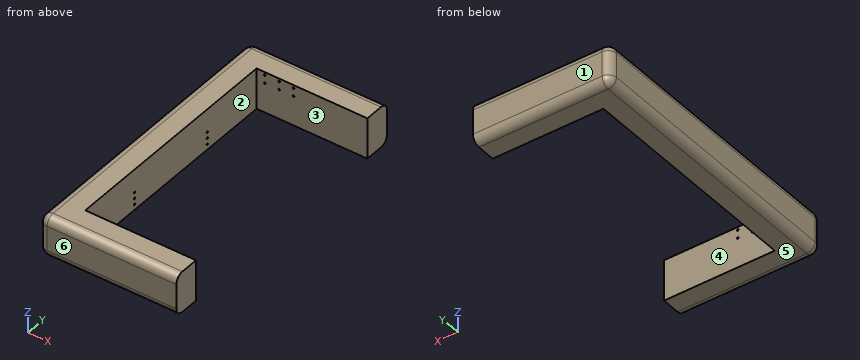
Autodesk Inventor part; units mm, degrees
ref_plane "YZ Plane" through (0, 0, 0) normal (1, 0, 0) x (0, 1, 0)
ref_plane "XZ Plane" through (0, 0, 0) normal (0, 1, 0) x (-1, 0, 0)
ref_plane "XY Plane" through (0, 0, 0) normal (0, 0, 1) x (1, 0, 0)
sketch "Sketch1" plane through (0, 0, 0) normal (0, 0, 1) x (1, 0, 0)
  line L0 (0, 0) -> (0, 719.074)
  line L1 (0, 719.074) -> (342.9, 719.074)
  line L2 (0, 0) -> (342.9, 0)
  line L3 (342.9, 801.624) -> (-82.55, 801.624)
  line L4 (-82.55, 801.624) -> (-82.55, -82.55)
  line L5 (-82.55, -82.55) -> (342.9, -82.55)
  line L6 (342.9, 719.074) -> (342.9, 801.624)
  line L7 (342.9, 0) -> (342.9, -82.55)
  dimension "d0" = 719.074
  dimension "d1" = 342.9
  dimension "d2" = 82.55
extrude "Extrusion1" add sketch "Sketch1" along normal blind 127
fillet "Fillet1" radius 25.4 8 edges at (130.175, 801.624, 127) (130.175, 801.624, 0) (-82.55, 801.624, 63.5) (-82.55, 359.537, 127) (-82.55, 359.537, 0) (-82.55, -82.55, 63.5) (130.175, -82.55, 0) (130.175, -82.55, 127)
sketch "Sketch2" plane through (0, 719.074, 0) normal (0, -1, 0) x (1, 0, 0)
  line L0 (342.9, 0) -> (342.9, 127) construction
  line L1 (0, 127) -> (342.9, 127) construction
  line L2 (342.9, 127) -> (114.3, 127) construction
  line L3 (114.3, 127) -> (69.85, 127) construction
  line L4 (69.85, 127) -> (25.4, 127) construction
  line L5 (114.3, 127) -> (114.3, 117.475) construction
  line L6 (114.3, 117.475) -> (69.85, 117.475) construction
  line L7 (69.85, 117.475) -> (25.4, 117.475) construction
  line L8 (25.4, 117.475) -> (25.4, 92.075) construction
  line L9 (25.4, 92.075) -> (69.85, 92.075) construction
  line L10 (69.85, 92.075) -> (114.3, 92.075) construction
  circle A0 centre (114.3, 117.475) radius 2.667
  circle A1 centre (69.85, 117.475) radius 2.667
  circle A2 centre (25.4, 117.475) radius 2.667
  circle A3 centre (25.4, 92.075) radius 2.667
  circle A4 centre (69.85, 92.075) radius 2.667
  circle A5 centre (114.3, 92.075) radius 2.667
  point P0 (0, 0)
  dimension "d7" = 228.6
  dimension "d8" = 44.45
  dimension "d9" = 44.45
  dimension "d10" = 9.525
  dimension "d11" = 25.4
  dimension "d12" = 5.334
extrude "Extrusion2" cut sketch "Sketch2" against normal blind 4.7625
sketch "Sketch3" plane through (0, 0, 0) normal (0, 1, 0) x (1, 0, 0)
  line L0 (342.9, -127) -> (0, -127) construction
  line L1 (342.9, -127) -> (342.9, -117.475) construction
  line L2 (342.9, 0) -> (342.9, -127) construction
  line L3 (342.9, -117.475) -> (114.3, -117.475) construction
  line L4 (114.3, -117.475) -> (69.85, -117.475) construction
  line L5 (69.85, -117.475) -> (25.4, -117.475) construction
  line L6 (25.4, -117.475) -> (25.4, -92.075) construction
  line L7 (25.4, -92.075) -> (69.85, -92.075) construction
  line L8 (69.85, -92.075) -> (114.3, -92.075) construction
  circle A0 centre (114.3, -117.475) radius 2.667
  circle A1 centre (69.85, -117.475) radius 2.667
  circle A2 centre (25.4, -117.475) radius 2.667
  circle A3 centre (25.4, -92.075) radius 2.667
  circle A4 centre (69.85, -92.075) radius 2.667
  circle A5 centre (114.3, -92.075) radius 2.667
  point P0 (0, 0)
  dimension "d15" = 9.525
  dimension "d16" = 228.6
  dimension "d17" = 44.45
  dimension "d18" = 44.45
  dimension "d19" = 25.4
  dimension "d20" = 5.334
extrude "Extrusion3" cut sketch "Sketch3" against normal blind 4.7625
sketch "Sketch4" plane through (0, 0, 0) normal (1, 0, 0) x (0, 0, -1)
  line L0 (-127, -57.15) -> (-127, 0) construction
  line L1 (-127, 0) -> (-127, 207.137) construction
  line L2 (-127, 0) -> (-127, 719.074) construction
  line L3 (-127, 207.137) -> (-55.118, 207.137) construction
  line L4 (-55.118, 207.137) -> (-36.068, 207.137) construction
  line L5 (-36.068, 207.137) -> (-17.018, 207.137) construction
  circle A0 centre (-55.118, 207.137) radius 2.667
  circle A1 centre (-36.068, 207.137) radius 2.667
  circle A2 centre (-17.018, 207.137) radius 2.667
  line L6 (-127, 359.537) -> (0, 359.537) construction
  line L7 (0, 0) -> (0, 719.074) construction
  line L8 (-55.118, 511.937) -> (-36.068, 511.937) construction
  line L9 (-36.068, 511.937) -> (-17.018, 511.937) construction
  circle A3 centre (-55.118, 511.937) radius 2.667
  circle A4 centre (-36.068, 511.937) radius 2.667
  circle A5 centre (-17.018, 511.937) radius 2.667
  dimension "d23" = 207.137
  dimension "d24" = 71.882
  dimension "d25" = 19.05
  dimension "d26" = 19.05
  dimension "d27" = 5.334
extrude "Extrusion4" cut sketch "Sketch4" against normal blind 4.7625
properties part number "Bumper Side"
Work out the finished part from the listing and answer in its coordinate system (mm). Face numbers are marked on the shaded views. A direction names the side the tool comes from. Round coordinates to 2 decimals unless told otherwise and drop trailing zeros. Loops run counter-clockwise (first coordinate to the right, second up) from the corner with the lowest first, then second, coordinate; pieces in that order, holes last. Notation, with made-up numbers: (42.25, 6) - (94.25, 6) arc R15 ccw to (94.25, 32) - close; hole circle Ø2 at (-4, 63.5). An arc over 180 degrees is marked (long way). Use one line per item in the form item = value. Start each with the question number.
(1) Find section A-A on x = 13. Determine the outline of the cut face in (y, z), and give its area (3 significant figures).
(2) Which of the six approach directions +Z, -Z, +X, -X, +Y, -Y give full straight-line access (tool end or side, diameter ignored) to the marked faces 1 and 2?
(3) Flat-ended cylindrical pins translate along their axes: P1, Ø3, axis at x = 281, z = 22.5, coming from the -Y side; P2, Ø2, axis at x = 16, z = 21.5, coming from the -Y side; P3, Ø1.6, axis at x = 113.5, z = 118.5, coming from the +Y side. Find the tip coordinate at first contact, or state that the pin passes through.
(4) Determine the mould class of the marked faces 3, 4, 5 and 6 for opening direction Y: +Y half, -Y half, draft (parallel to the pull), parting line (faces both ways), or undercut.
(5) Find section B-B on y = 409. Determine the outline of the cut face in (x, z), and give its area (3 significant figures).
(6) Consider line 1 (Z direction, x = 25.4, y = -3.2); line 2 (Z direction, x = 69, y = 722); line 3 (Y direction, x = 38.5, z = 33). Determine where each line is inside the solid, lowest interval first.
Answer list:
q1.outline = (-82.55, 25.4) arc R25.4 ccw to (-57.15, 0) - (0, 0) - (0, 127) - (-57.15, 127) arc R25.4 ccw to (-82.55, 101.6) - close; (719.07, 0) - (776.22, 0) arc R25.4 ccw to (801.62, 25.4) - (801.62, 101.6) arc R25.4 ccw to (776.22, 127) - (719.07, 127) - close
q1.area = 20,400 mm^2
q2.face_1 = +Z, -Z, +X, -X, +Y
q2.face_2 = +Z, -Z, +X
q3.P1 = -82.51
q3.P2 = -82.38
q3.P3 = 795.87
q4.face_3 = undercut
q4.face_4 = undercut
q4.face_5 = draft
q4.face_6 = -Y half
q5.outline = (-82.55, 25.4) arc R25.4 ccw to (-57.15, 0) - (0, 0) - (0, 127) - (-57.15, 127) arc R25.4 ccw to (-82.55, 101.6) - close
q5.area = 10,200 mm^2
q6.line_1 = 0 to 89.41, 94.74 to 114.81, 120.14 to 127
q6.line_2 = 0 to 89.55, 94.6 to 114.95, 120 to 127
q6.line_3 = -82.55 to 0, 719.07 to 801.62
